Can you work these out from the model? Positions are in its coordinate system, mm. A direction names the side the tool comes from. Round coordinates to 2 decimals unless told otherwise and drop trailing zeros. Loops run counter-clockwise (first coordinate to the right, second up) from the corner with the lowest first, then second, coordinate; pieces in that order, holes last. Notation, with made-up numbers: (-5, 51) -> (28, 51) arc R17 ccw to (28, 84) -> close; hole circle Ø11 at (60, 86). An arc over 180 degrees is marked (long way). Write each question's results on one line, items separated by ' | '.
from build123d import *

# Parameters (mm, degrees)
F0_R      = 19.05
F1_DEPTH  = 63.5
F2_W      = 50.8
F2_H      = 36.4998
F3_DEPTH  = 63.501
F5_DEPTH  = 63.501
F6_R      = 5.5626
F7_DEPTH  = 20.6502
F8_DEPTH  = 20.6512
F9_DEPTH  = 25.4
F10_DEPTH = 25.4


with BuildPart() as f1:
    # F0 (on Front) → F1 (new body)
    with BuildSketch(Plane.XZ):
        with BuildLine():
            Line((84.1502, 28.575), (0, 28.575))
            ThreePointArc((0, 28.575), (-28.575, 0), (0, -28.575))
            Line((0, -28.575), (84.1502, -28.575))
            Line((84.1502, -28.575), (84.1502, 28.575))
        make_face()
        Circle(F0_R, mode=Mode.SUBTRACT)
    extrude(amount=-F1_DEPTH)

    # F2 (on Front) → F3 (cut, through all)
    with BuildSketch(Plane.XZ):
        with Locations((58.7502, -10.3251)):
            Rectangle(F2_W, F2_H)
    extrude(amount=-F3_DEPTH, mode=Mode.SUBTRACT)

    # F4 (on Front) → F5 (cut, through all)
    with BuildSketch(Plane.XZ):
        with BuildLine():
            ThreePointArc((28.575, 0), (20.205576, -20.205576), (0, -28.575))
            Line((0, -28.575), (33.3502, -28.575))
            Line((33.3502, -28.575), (33.3502, 7.9248))
            Line((33.3502, 7.9248), (28.575, 7.9248))
            Line((28.575, 7.9248), (28.575, 0))
        make_face()
    extrude(amount=-F5_DEPTH, mode=Mode.SUBTRACT)

    # F6 (on face) → F7 (join)
    with BuildSketch(Plane(origin=(0, 0, 7.9248), x_dir=(1, 0, 0), z_dir=(0, 0, -1))):
        with BuildLine():
            ThreePointArc((84.1502, -37.3126), (78.5876, -31.75), (84.1502, -26.1874))
            Line((84.1502, -26.1874), (84.1502, -17.124132))
            Line((84.1502, -17.124132), (57.099155, -1.672279))
            ThreePointArc((57.099155, -1.672279), (54.058676, -0.425187), (50.8, 0))
            ThreePointArc((50.8, 0), (41.819744, -3.719744), (38.1, -12.7))
            Line((38.1, -12.7), (38.1, -50.8))
            ThreePointArc((38.1, -50.8), (41.819744, -59.780256), (50.8, -63.5))
            ThreePointArc((50.8, -63.5), (54.058676, -63.074813), (57.099155, -61.827721))
            Line((57.099155, -61.827721), (84.1502, -46.375868))
            Line((84.1502, -46.375868), (84.1502, -37.3126))
        make_face()
        with Locations((50.8, -50.8)):
            Circle(F6_R, mode=Mode.SUBTRACT)
        with Locations((50.8, -12.7)):
            Circle(F6_R, mode=Mode.SUBTRACT)
        with BuildLine():
            ThreePointArc((84.1502, -26.1874), (88.083552, -27.816648), (89.7128, -31.75))
            ThreePointArc((89.7128, -31.75), (88.083552, -35.683352), (84.1502, -37.3126))
            Line((84.1502, -37.3126), (84.1502, -46.375868))
            Line((84.1502, -46.375868), (90.449355, -42.777721))
            ThreePointArc((90.449355, -42.777721), (96.8502, -31.75), (90.449355, -20.722279))
            Line((90.449355, -20.722279), (84.1502, -17.124132))
            Line((84.1502, -17.124132), (84.1502, -26.1874))
        make_face()
    extrude(amount=-F7_DEPTH)

    # F6 (on face) → F8 (cut, through all)
    with BuildSketch(Plane(origin=(0, 0, 7.9248), x_dir=(1, 0, 0), z_dir=(0, 0, -1))):
        with Locations((50.8, -12.7)):
            Circle(F6_R)
        with Locations((50.8, -50.8)):
            Circle(F6_R)
        with BuildLine():
            Line((84.1502, -37.3126), (84.1502, -26.1874))
            ThreePointArc((84.1502, -26.1874), (78.5876, -31.75), (84.1502, -37.3126))
        make_face()
    extrude(amount=-F8_DEPTH, mode=Mode.SUBTRACT)

    # F6 (on face) → F9 (cut)
    with BuildSketch(Plane(origin=(0, 0, 7.9248), x_dir=(1, 0, 0), z_dir=(0, 0, -1))):
        with BuildLine():
            Line((57.099155, -1.672279), (84.1502, -17.124132))
            Line((84.1502, -17.124132), (84.1502, 0))
            Line((84.1502, 0), (50.8, 0))
            ThreePointArc((50.8, 0), (54.058676, -0.425187), (57.099155, -1.672279))
        make_face()
        with BuildLine():
            Line((84.1502, -63.5), (84.1502, -46.375868))
            Line((84.1502, -46.375868), (57.099155, -61.827721))
            ThreePointArc((57.099155, -61.827721), (54.058676, -63.074813), (50.8, -63.5))
            Line((50.8, -63.5), (84.1502, -63.5))
        make_face()
    extrude(amount=-F9_DEPTH, mode=Mode.SUBTRACT)

    # F6 (on face) → F10 (join)
    with BuildSketch(Plane(origin=(0, 0, 7.9248), x_dir=(1, 0, 0), z_dir=(0, 0, -1))):
        with BuildLine():
            ThreePointArc((84.1502, -37.3126), (78.5876, -31.75), (84.1502, -26.1874))
            Line((84.1502, -26.1874), (84.1502, -17.124132))
            Line((84.1502, -17.124132), (57.099155, -1.672279))
            ThreePointArc((57.099155, -1.672279), (54.058676, -0.425187), (50.8, 0))
            ThreePointArc((50.8, 0), (41.819744, -3.719744), (38.1, -12.7))
            Line((38.1, -12.7), (38.1, -50.8))
            ThreePointArc((38.1, -50.8), (41.819744, -59.780256), (50.8, -63.5))
            ThreePointArc((50.8, -63.5), (54.058676, -63.074813), (57.099155, -61.827721))
            Line((57.099155, -61.827721), (84.1502, -46.375868))
            Line((84.1502, -46.375868), (84.1502, -37.3126))
        make_face()
        with Locations((50.8, -50.8)):
            Circle(F6_R, mode=Mode.SUBTRACT)
        with Locations((50.8, -12.7)):
            Circle(F6_R, mode=Mode.SUBTRACT)
        with BuildLine():
            ThreePointArc((84.1502, -26.1874), (88.083552, -27.816648), (89.7128, -31.75))
            ThreePointArc((89.7128, -31.75), (88.083552, -35.683352), (84.1502, -37.3126))
            Line((84.1502, -37.3126), (84.1502, -46.375868))
            Line((84.1502, -46.375868), (90.449355, -42.777721))
            ThreePointArc((90.449355, -42.777721), (96.8502, -31.75), (90.449355, -20.722279))
            Line((90.449355, -20.722279), (84.1502, -17.124132))
            Line((84.1502, -17.124132), (84.1502, -26.1874))
        make_face()
    extrude(amount=-F10_DEPTH)


solid = f1.part
1. If we section it at A-A (y = 36): List the corners of the cut face in (x, z) for me (3 decimals), then the cut area to 3 significant figures.
Final values:
outline: (0, 28.575) arc R28.575 ccw (long way) to (28.575, 0) -> (28.575, 7.925) -> (80.561, 7.925) -> (80.561, 33.325) -> (38.1, 33.325) -> (38.1, 28.575) -> close; (87.739, 7.925) -> (96.118, 7.925) -> (96.118, 33.325) -> (87.739, 33.325) -> close; hole circle Ø38.1 at (0, 0) | area: 3,090 mm2
2. If we section it at D-D (z = 20.5): List the corners of the cut face in (x, y) for me, then the cut area to 3 significant figures.
Final values:
outline: (-19.91, 0) -> (50.8, 0) arc R12.7 ccw to (57.1, 1.67) -> (90.45, 20.72) arc R12.7 ccw to (90.45, 42.78) -> (57.1, 61.83) arc R12.7 ccw to (50.8, 63.5) -> (-19.91, 63.5) -> close; hole circle Ø11.13 at (50.8, 12.7); hole circle Ø11.13 at (50.8, 50.8); hole (84.15, 37.31) arc R5.56 ccw (long way) to (89.71, 31.75) arc R5.56 ccw to start | area: 6,060 mm2
3. Will these pins go through, and if not, where does the flat tip stop? pin 1 (6.5 mm diameter, centred on y = 22, z = 3.5, fed in from +X) (3 decimals); pin 2 (3 mm diameter, centred on x = 61.5, y = 7, fed in from -Z); pin 3 (1.4 mm diameter, centred on y = 39, z = 32, fed in from -X); pin 4 (14.5 mm diameter, centred on x = 50.8, y = 12.7, fed in from +Z).
Final values:
pin 1: x = 28.575 | pin 2: z = 7.92 | pin 3: x = 38.1 | pin 4: z = 33.32
4. Please list where these lines run through material, in increasing order: line 1 (Y direction, x = 50.8, z = 27.5); line 2 (Z direction, x = 0, y = 47) (3 decimals); line 3 (X direction, y = 10, z = -6). Write a range as from..to.
Final values:
line 1: 0..7.14, 18.26..45.24, 56.36..63.5 | line 2: -28.575..-19.05, 19.05..28.575 | line 3: -27.94..-18.08, 18.08..27.94
5. If we section it at C-C (z = -17): List the corners of the cut face in (x, y) for me, then the cut area to 3 significant figures.
Final values:
outline: (-22.97, 0) -> (-8.6, 0) -> (-8.6, 63.5) -> (-22.97, 63.5) -> close; (8.6, 0) -> (22.97, 0) -> (22.97, 63.5) -> (8.6, 63.5) -> close | area: 1,830 mm2
6. If we section it at B-B (z = 13): List the corners of the cut face in (x, y) for me.
Final values:
outline: (-25.45, 0) -> (-13.92, 0) -> (-13.92, 63.5) -> (-25.45, 63.5) -> close; (13.92, 0) -> (50.8, 0) arc R12.7 ccw to (57.1, 1.67) -> (90.45, 20.72) arc R12.7 ccw to (90.45, 42.78) -> (57.1, 61.83) arc R12.7 ccw to (50.8, 63.5) -> (13.92, 63.5) -> close; hole circle Ø11.13 at (50.8, 12.7); hole circle Ø11.13 at (50.8, 50.8); hole (84.15, 37.31) arc R5.56 ccw (long way) to (89.71, 31.75) arc R5.56 ccw to start
7. On a 3-axis mill with a long thin cutter (end or side, diameter ignored), from which of +Z, -Z, +X, -X, +Y, -Y can I reach the whole of each face in a straight line? I mean faces 1 (the face through (41.92, 3.62, 30.92)), 2 (the face through (38.1, 31, 31)), 3 (the face through (41.72, 59.68, 30.92)), 4 (the face through (55, 31, 7.925)). Say none if no direction works.
Final values:
face 1: +Z, -X, -Y | face 2: +Z, -X, +Y, -Y | face 3: +Z, -X, +Y | face 4: -Z, +X, +Y, -Y
8. We'd pull the mould along Z, two halves only. Please class faces 5 (the face through (19, 63.5, 7)), 6 (the face through (-15.12, 31.31, -11.59)), 7 (the face through (61, 31, 33.325)): pulls with the +Z half, pulls with the -Z half, needs draft (parallel to the pull), parting line crosses it, or undercut.
Final values:
face 5: needs draft | face 6: undercut | face 7: pulls with the +Z half
